```python
from build123d import *

# Parameters (mm, degrees)
SKETCH1_R               = 18.3
BOSS_EXTRUDE1_DEPTH     = 19.2
SKETCH2_R               = 1.6
CUT_EXTRUDE1_DEPTH      = 3.5
SKETCH3_R               = 3
BOSS_EXTRUDE2_DEPTH     = 35
SKETCH3_3_R             = 6
SKETCH3_3_R_2           = 3
BOSS_EXTRUDE3_DEPTH     = 4
SKETCH4_R               = 13.8
BOSS_EXTRUDE4_DEPTH     = 33.5
SKETCH5_R               = 5
BOSS_EXTRUDE5_DEPTH     = 3
SKETCH6_R               = 1
BOSS_EXTRUDE6_DEPTH     = 5
SKETCH7_W               = 0.5
SKETCH7_H               = 3
BOSS_EXTRUDE7_DEPTH     = 6.5
CUT_EXTRUDE2_DEPTH      = 0.5
FILLET1_R               = 0.5
CHAMFER1_SIZE           = 0.2
SKETCH9_R               = 1.6
CUT_EXTRUDE3_DEPTH      = 12.3
CUT_EXTRUDE3_DEPTH_BACK = 26.3


with BuildPart() as part:
    # Sketch1 → Boss-Extrude1 (new body)
    with BuildSketch(Plane.XY):
        Circle(SKETCH1_R)
    extrude(amount=BOSS_EXTRUDE1_DEPTH)

    # Sketch2 → Cut-Extrude1 (cut)
    with BuildSketch(Plane.XY.offset(19.2)):
        with Locations((-7.75, 13.423393759)):
            Circle(SKETCH2_R)
        with Locations((7.75, 13.423393759)):
            Circle(SKETCH2_R)
        with Locations((-15.5, 0)):
            Circle(SKETCH2_R)
        with Locations((-7.75, -13.423393759)):
            Circle(SKETCH2_R)
        with Locations((7.75, -13.423393759)):
            Circle(SKETCH2_R)
        with Locations((15.5, 0)):
            Circle(SKETCH2_R)
    extrude(amount=-CUT_EXTRUDE1_DEPTH, mode=Mode.SUBTRACT)

    # Sketch3 → Boss-Extrude2 (add)
    with BuildSketch(Plane.XY.offset(19.2)):
        with Locations((0, 7)):
            Circle(SKETCH3_R)
    extrude(amount=BOSS_EXTRUDE2_DEPTH)

    # Sketch3<3> → Boss-Extrude3 (add)
    with BuildSketch(Plane.XY.offset(19.2)):
        with Locations((0, 7)):
            Circle(SKETCH3_3_R)
        with Locations((0, 7)):
            Circle(SKETCH3_3_R_2, mode=Mode.SUBTRACT)
    extrude(amount=BOSS_EXTRUDE3_DEPTH)

    # Sketch4 → Boss-Extrude4 (add)
    with BuildSketch(Plane(origin=(0, 0, 0), x_dir=(-1, 0, 0), z_dir=(0, 0, -1))):
        Circle(SKETCH4_R)
    extrude(amount=BOSS_EXTRUDE4_DEPTH)

    # Sketch5 → Boss-Extrude5 (add)
    with BuildSketch(Plane(origin=(0, 0, -33.5), x_dir=(-1, 0, 0), z_dir=(0, 0, -1))):
        Circle(SKETCH5_R)
    extrude(amount=BOSS_EXTRUDE5_DEPTH)

    # Sketch6 → Boss-Extrude6 (add)
    with BuildSketch(Plane(origin=(0, 0, -36.5), x_dir=(-1, 0, 0), z_dir=(0, 0, -1))):
        Circle(SKETCH6_R)
    extrude(amount=BOSS_EXTRUDE6_DEPTH)

    # Sketch7 → Boss-Extrude7 (add)
    with BuildSketch(Plane(origin=(0, 0, -33.5), x_dir=(-1, 0, 0), z_dir=(0, 0, -1))):
        with Locations((-11.75, 0)):
            Rectangle(SKETCH7_W, SKETCH7_H)
        with Locations((11.75, 0)):
            Rectangle(SKETCH7_W, SKETCH7_H)
    extrude(amount=BOSS_EXTRUDE7_DEPTH)

    # Sketch8 → Cut-Extrude2 (cut)
    with BuildSketch(Plane(origin=(12, 0, 0), x_dir=(0, 0, -1), z_dir=(1, 0, 0))):
        with BuildLine():
            Line((38.1, -0.4), (36.9, -0.4))
            ThreePointArc((36.9, -0.4), (36.5, 0), (36.9, 0.4))
            Line((36.9, 0.4), (38.1, 0.4))
            ThreePointArc((38.1, 0.4), (38.5, 0), (38.1, -0.4))
        make_face()
    cut_extrude2 = extrude(amount=-CUT_EXTRUDE2_DEPTH, mode=Mode.SUBTRACT)

    # Mirror2: Cut-Extrude2 across plane
    add(cut_extrude2.mirror(Plane(origin=(0, 0, 0), x_dir=(0, 0, 1), z_dir=(1, 0, 0))), mode=Mode.SUBTRACT)

    # Fillet1
    fillet1_edges = [part.edges().sort_by_distance(p)[0] for p in [
        (11.75, -1.5, -40),
        (11.75, 1.5, -40),
        (-11.75, 1.5, -40),
        (-11.75, -1.5, -40),
    ]]
    fillet(fillet1_edges, radius=FILLET1_R)

    # Chamfer1
    chamfer1_edges = [part.edges().sort_by_distance(p)[0] for p in [
        (-3, 7, 54.2),
        (-6, 7, 23.2),
        (-18.3, 0, 19.2),
    ]]
    chamfer(chamfer1_edges, length=CHAMFER1_SIZE)

    # Sketch9 → Cut-Extrude3 (cut, two sides)
    with BuildSketch(Plane(origin=(0, 7, 0), x_dir=(1, 0, 0), z_dir=(0, 1, 0))) as cut_extrude3_sk:
        with Locations((0, -46.2)):
            Circle(SKETCH9_R)
    extrude(amount=CUT_EXTRUDE3_DEPTH, mode=Mode.SUBTRACT)
    extrude(cut_extrude3_sk.sketch, amount=-CUT_EXTRUDE3_DEPTH_BACK, mode=Mode.SUBTRACT)


solid = part.part
```
Verification items for the finished model (mm, model axes). A direction names the side the tool comes from. Give positions to 0.01 mm unless a question says otherwise; leave off trailing zeros. Order: outer loops, then holes, each group sorted by start corner. A loop starts at its lowest first (then second) coordinate and runs counter-clockwise, first axis right, second up. Notation, with made-up numbers: (65.25, 74.5) - (124.25, 74.5) arc R22 cw to (124.25, 97.5) - close; hole circle Ø1 at (31, -25). An arc over 180 degrees is marked (long way). Answer as CSV lines item,"result". Start each with the question number.
Item 1: Gauge pin test, flat ends, axial feed: pin 1 (5 mm diameter, centred on x = 2, y = -5, fed in from -Z); pin 2 (8 mm diameter, centred on x = 13.5, y = 1.5, fed in from +Z); pin 3 (3 mm diameter, centred on x = -11, y = 0.5, fed in from -Z). Record the tip position at first contact, or that the pin passes through.
Item 2: Mould release check, pull along X, two halves, no side actions. Record for faces 1 (the face through (2.86, 7.9, 38.38)), 2 (the face through (12, 0, -36)), 3 (the face through (2.5, 4.5, 23.2)), 4 (the face through (-16, 0, 15.7)): released by +X, released by -X, zero draft, split by the parting line, or undercut.
Item 3: Section check C-C, the plane z = -10.5. Record the boundary of the cut face in (x, y).
Item 4: Access from +Z, -Z, +X, -X, +Y, -Y to the whole of each face (thin tool, end or side, straight path). Record for faces 5 (the face through (3, 14, 0)), 6 (the face through (0, 0, -41.5)), 7 (the face through (-7.96, 15.01, 17.47)).
Item 5: Material ranges on L1, parallel to Z at x = 0, y = 8; L2, parallel to Y at x = 7.75, z = 17.8; L3, parallel to Y at x = -7, z = 18, recorded low to high.
Item 6: Section check B-B, the plane z = 17.5. Record the boundary of the cut face in (x, y).
Filled in:
1,pin 1,"z = -36.5"
1,pin 2,"z = 19.2"
1,pin 3,"z = -40"
2,face 1,"split by the parting line"
2,face 2,"released by +X"
2,face 3,"zero draft"
2,face 4,"undercut"
3,outline,"circle Ø27.6 at (0, 0)"
4,face 5,"-Z"
4,face 6,"-Z, +X, -X, +Y, -Y"
4,face 7,"+Z"
5,L1,"-33.5 to 44.6, 47.8 to 54.2"
5,L2,"-16.58 to -15.02, -11.82 to 11.82, 15.02 to 16.58"
5,L3,"-16.91 to -14.84, -12.01 to 12.01, 14.84 to 16.91"
6,outline,"circle Ø36.6 at (0, 0); hole circle Ø3.2 at (-15.5, 0); hole circle Ø3.2 at (-7.75, -13.42); hole circle Ø3.2 at (-7.75, 13.42); hole circle Ø3.2 at (7.75, -13.42); hole circle Ø3.2 at (7.75, 13.42); hole circle Ø3.2 at (15.5, 0)"
